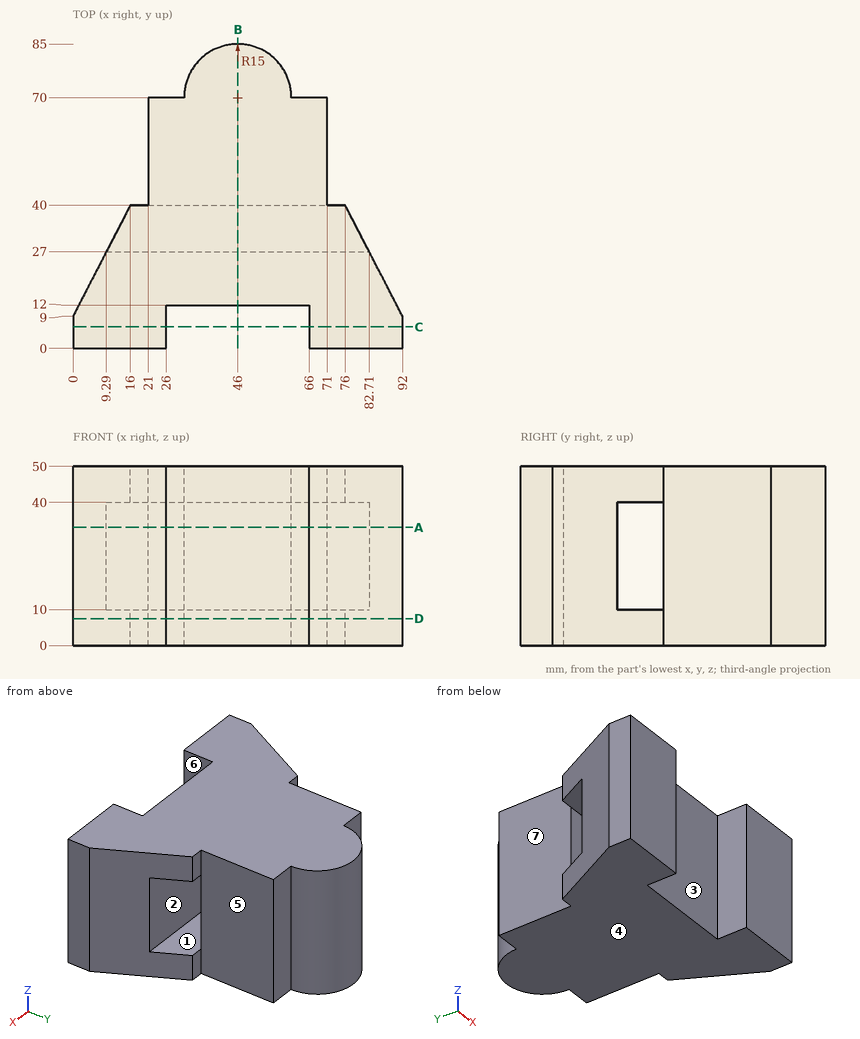
Source: three-view drawing plus pictorial views. Frame: mm from the lowest corner of the part. A direction names the side the tool comes from. Give positions to 0.01 mm unless a question says otherwise; leave off trailing zeros. Loops run counter-clockwise (first coordinate to the right, second up) from the corner with the lowest first, then second, coordinate; pieces in that order, holes last.
1) Reachability of the marked faces 5, 6 and 7 from +Z, -Z, +X, -X, +Y, -Y: full face, straight path, thin tool, end or side. Return the list, or none.
A:
face 5: +Z, -Z, +X, +Y
face 6: +Z, -Z, -Y
face 7: +Z, -Z, -X, +Y
2) Contact query for flat-ended pins moving along their axis: pin 1 (15 mm diameter, centred on y = 55.5, z = 28, fed in from -X); pin 2 (10 mm diameter, centred on y = 27, z = 41.5, fed in from +X); pin 3 (5.5 mm diameter, centred on x = 19, z = 46, fed in from +Y); pin 4 (6 mm diameter, centred on x = 37, y = 8.5, fed in from -Z). Output: stop coordinate, or through.
A:
pin 1: stops at x = 21
pin 2: stops at x = 85.29
pin 3: stops at y = 70
pin 4: passes through
3) Section query D-D on z = 7.5. Return the cut outline in (x, y).
A:
outline: (0, 0) - (26, 0) - (26, 12) - (66, 12) - (66, 0) - (92, 0) - (92, 9) - (76, 40) - (71, 40) - (71, 70) - (61, 70) arc R15 ccw to (31, 70) - (21, 70) - (21, 40) - (16, 40) - (0, 9) - close
4) Section query B-B on x = 46. Return the cut outline in (y, z).
A:
outline: (12, 0) - (85, 0) - (85, 50) - (12, 50) - close; hole (27, 10) - (40, 10) - (40, 40) - (27, 40) - close
5) Section query C-C on y = 6. Return the cut outline in (x, z), and give its area (3 significant figures).
A:
outline: (0, 0) - (26, 0) - (26, 50) - (0, 50) - close; (66, 0) - (92, 0) - (92, 50) - (66, 50) - close
area: 2,600 mm2
6) Mould query, pull axis Z, two halves, no side actions, for the marked faces 1, 2, 3 and 4. Classes: released by +Z, released by -Z, zero draft, split by the parting line, or undercut.
A:
face 1: undercut
face 2: undercut
face 3: zero draft
face 4: released by -Z
7) Section query A-A on z = 33. Return the cut outline in (x, y), and give its area (3 significant figures).
A:
outline: (0, 0) - (26, 0) - (26, 12) - (66, 12) - (66, 0) - (92, 0) - (92, 9) - (82.71, 27) - (9.29, 27) - (0, 9) - close; (21, 40) - (71, 40) - (71, 70) - (61, 70) arc R15 ccw to (31, 70) - (21, 70) - close
area: 3,690 mm2
8) Line query: L1, parallel to Y at x = 30, z = 17; L2, parallel to X at y = 52.5, z = 33; L3, parallel to Y at x = 72.5, z = 44.5. Output: solid intervals per line, ascending.
A:
L1: y = 12 to 27, 40 to 70
L2: x = 21 to 71
L3: y = 0 to 40
